Could you check a few things on this drawing? It's one solid part, dimensions in mm from its lowest x, y, z. A direction names the side the tool comes from. Coordinates: 2 decimals unless noted, no trailing zeros. Order: outer loops, then holes, each group sorted by start corner. A loop starts at its lowest first (then second) coordinate and runs counter-clockwise, first axis right, second up.
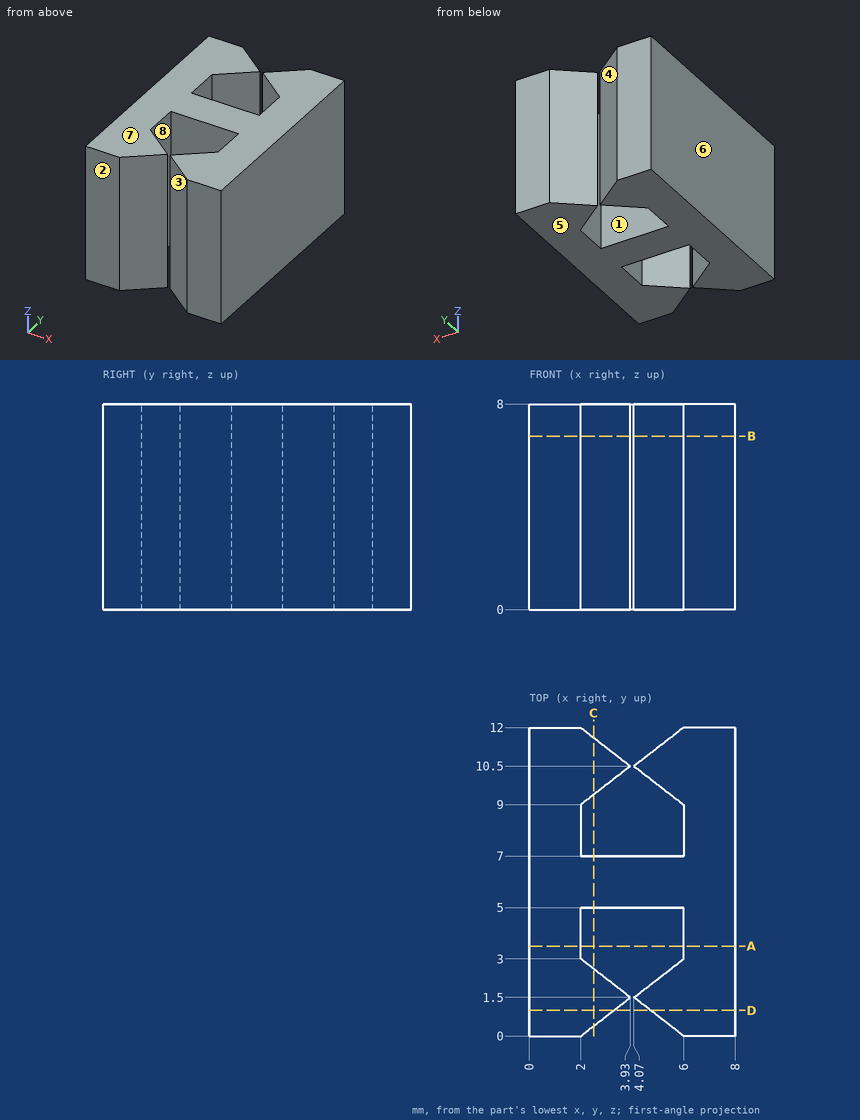
Item 1: Suppose I cut it at B-B (z = 6.75). List the corners of the cut face in (x, y) for me.
Item 2: For pin 1 Ø1 at (y, z) = (7.5, 2.5) entering from -X; pin 2 Ø1.2 at (x, z) = (4, 3) entering from -Y, each with a flat end and sliding along its axis, tell me the tip position at first contact or that it passes through.
Item 3: Suppose I cut it at C-C (x = 2.5). List the corners of the cut face in (y, z) for me, and give its area (3 significant figures).
Item 4: Suppose I cut it at D-D (y = 1). List the corners of the cut face in (x, z) for me.
Item 5: Which directions (+Z, -Z, +X, -X, +Y, -Y) give clear straight access to the entire face, cutting with the end or side of a thin tool? Please do the marked faces 1, 2, 3, 4 and 5.
Item 6: I need wall thicknesses on line 1 (X direction, y = 7.75, z = 2); line 2 (Y direction, x = 3, z = 6); line 3 (X direction, y = 1, z = 5). Which ranges of each line are inside material? Lowest first, please.
Item 7: Suppose I cut it at A-A (y = 3.5). List the corners of the cut face in (x, z) for me.
Item 8: Thinking about a two-plate mould opening in X: for the marked faces 6, 7 and 8, which applies, +X half, -X half, draft (parallel to the pull), parting line (faces both ways), or undercut?
Geometry results:
1. outline: (0, 0) - (2, 0) - (3.93, 1.5) - (2, 3) - (2, 5) - (6, 5) - (6, 3) - (4.07, 1.5) - (6, 0) - (8, 0) - (8, 12) - (6, 12) - (4.07, 10.5) - (6, 9) - (6, 7) - (2, 7) - (2, 9) - (3.93, 10.5) - (2, 12) - (0, 12) - close
2. pin 1: stops at x = 0
2. pin 2: stops at y = 1.09
3. outline: (0.39, 0) - (2.61, 0) - (2.61, 8) - (0.39, 8) - close; (5, 0) - (7, 0) - (7, 8) - (5, 8) - close; (9.39, 0) - (11.61, 0) - (11.61, 8) - (9.39, 8) - close
3. area: 51.6 mm2
4. outline: (0, 0) - (3.29, 0) - (3.29, 8) - (0, 8) - close; (4.71, 0) - (8, 0) - (8, 8) - (4.71, 8) - close
5. face 1: +Z, -Z
5. face 2: +Z, -Z, +X, -X, -Y
5. face 3: +Z, -Z, -Y
5. face 4: +Z, -Z, +Y
5. face 5: -Z, +X, -X, +Y, -Y
6. line 1: x = 0 to 2, 6 to 8
6. line 2: y = 0.78 to 2.22, 5 to 7, 9.78 to 11.22
6. line 3: x = 0 to 3.29, 4.71 to 8
7. outline: (0, 0) - (2, 0) - (2, 8) - (0, 8) - close; (6, 0) - (8, 0) - (8, 8) - (6, 8) - close
8. face 6: -X half
8. face 7: draft
8. face 8: undercut
